from build123d import *

# Parameters (mm, degrees)
SKETCH1_W           = 60
SKETCH1_H           = 45.5
SKETCH1_R           = 1.5
BOSS_EXTRUDE3_DEPTH = 1.6


with BuildPart() as part:
    # Sketch1 → Boss-Extrude3 (new body)
    with BuildSketch(Plane(origin=(0, 0, 0), x_dir=(1, 0, 0), z_dir=(0, 1, 0))):
        with Locations((0, 9.56004902)):
            Rectangle(SKETCH1_W, SKETCH1_H)
        with Locations(Location((-26, 28.31004902, 0), (0, 0, 270))):
            Circle(SKETCH1_R, mode=Mode.SUBTRACT)
        with Locations(Location((26, 28.31004902, 0), (0, 0, 270))):
            Circle(SKETCH1_R, mode=Mode.SUBTRACT)
        with Locations(Location((-26, -9.18995098, 0), (0, 0, 270))):
            Circle(SKETCH1_R, mode=Mode.SUBTRACT)
        with Locations(Location((26, -9.18995098, 0), (0, 0, 270))):
            Circle(SKETCH1_R, mode=Mode.SUBTRACT)
        with BuildLine():
            Line((-15.25, -8.18995098), (15.25, -8.18995098))
            ThreePointArc((15.25, -8.18995098), (0, 17.31004902), (-15.25, -8.18995098))
        make_face(mode=Mode.SUBTRACT)
    extrude(amount=BOSS_EXTRUDE3_DEPTH)


solid = part.part
Design review of the part built by this model. Coordinates are the model's own, in mm. Coordinates: 2 decimals unless noted, no trailing zeros. Loops run counter-clockwise (first coordinate to the right, second up) from the corner with the lowest first, then second, coordinate; pieces in that order, holes last. Notation, with made-up numbers: (55.5, 59) -> (65.5, 59) arc R21 cw to (65.5, 88) -> close; hole circle Ø3 at (58.25, 18.25). An arc over 180 degrees is marked (long way). Use a Markdown table: item, result. Add a question column.
Item 1: We need section C-C, the plane y = 1.05. Write out the cut boundary in (x, z).
Item 2: Wall thickness on L1, parallel to X at y = 1.1, z = -27; L2, parallel to X at y = 1.05, z = -7.5; L3, parallel to X at y = 0.6, z = -11: over which ranges is each line inside the solid? List them lowest first. Write a range as from..to.
Item 3: We need section A-A, the plane x = 0. Write out the cut boundary in (y, z), and give its area (3 significant figures).
Item 4: We need section D-D, the plane x = -26. Write out the cut boundary in (y, z), and give its area (3 significant figures).
Item 5: We need section B-B, the plane z = 0. Write out the cut boundary in (x, y).
Item 6: The part is to be moulded in two halves that separate along Z. For faces 1 (the cylindrical face through (27.487, 0.789, 8.995)), 2 (the flat face through (-30, 1, -9)), 3 (the flat face through (0, 1, 8.19)), 4 (the flat face through (0, 1, -32.31)), say which applies: +Z half, -Z half, draft (parallel to the pull), parting line (faces both ways), or undercut.
Numbers:
| question | item | result |
|---|---|---|
| 1 | outline | (-30, -32.31) -> (30, -32.31) -> (30, 13.19) -> (-30, 13.19) -> close; hole circle Ø3 at (-26, -28.31); hole circle Ø3 at (-26, 9.19); hole (-15.25, 8.19) arc R17.31 ccw (long way) to (15.25, 8.19) -> close; hole circle Ø3 at (26, -28.31); hole circle Ø3 at (26, 9.19) |
| 2 | L1 | x = -30..-26.73, -25.27..25.27, 26.73..30 |
| 2 | L2 | x = -30..-15.6, 15.6..30 |
| 2 | L3 | x = -30..-13.37, 13.37..30 |
| 3 | outline | (0, -32.31) -> (1.6, -32.31) -> (1.6, -17.31) -> (0, -17.31) -> close; (0, 8.19) -> (1.6, 8.19) -> (1.6, 13.19) -> (0, 13.19) -> close |
| 3 | area | 32.0 mm^2 |
| 4 | outline | (0, -32.31) -> (1.6, -32.31) -> (1.6, -29.81) -> (0, -29.81) -> close; (0, -26.81) -> (1.6, -26.81) -> (1.6, 7.69) -> (0, 7.69) -> close; (0, 10.69) -> (1.6, 10.69) -> (1.6, 13.19) -> (0, 13.19) -> close |
| 4 | area | 63.2 mm^2 |
| 5 | outline | (-30, 0) -> (-17.31, 0) -> (-17.31, 1.6) -> (-30, 1.6) -> close; (17.31, 0) -> (30, 0) -> (30, 1.6) -> (17.31, 1.6) -> close |
| 6 | face 1 | undercut |
| 6 | face 2 | draft |
| 6 | face 3 | undercut |
| 6 | face 4 | -Z half |
